Verification items for this drawing (mm, ordinates from the low corner). A direction names the side the tool comes from. Give positions to 0.01 mm unless a question says otherwise; leave off trailing zeros. Order: outer loops, then holes, each group sorted by start corner. A loop starts at its lowest first (then second) coordinate and runs counter-clockwise, first axis right, second up.
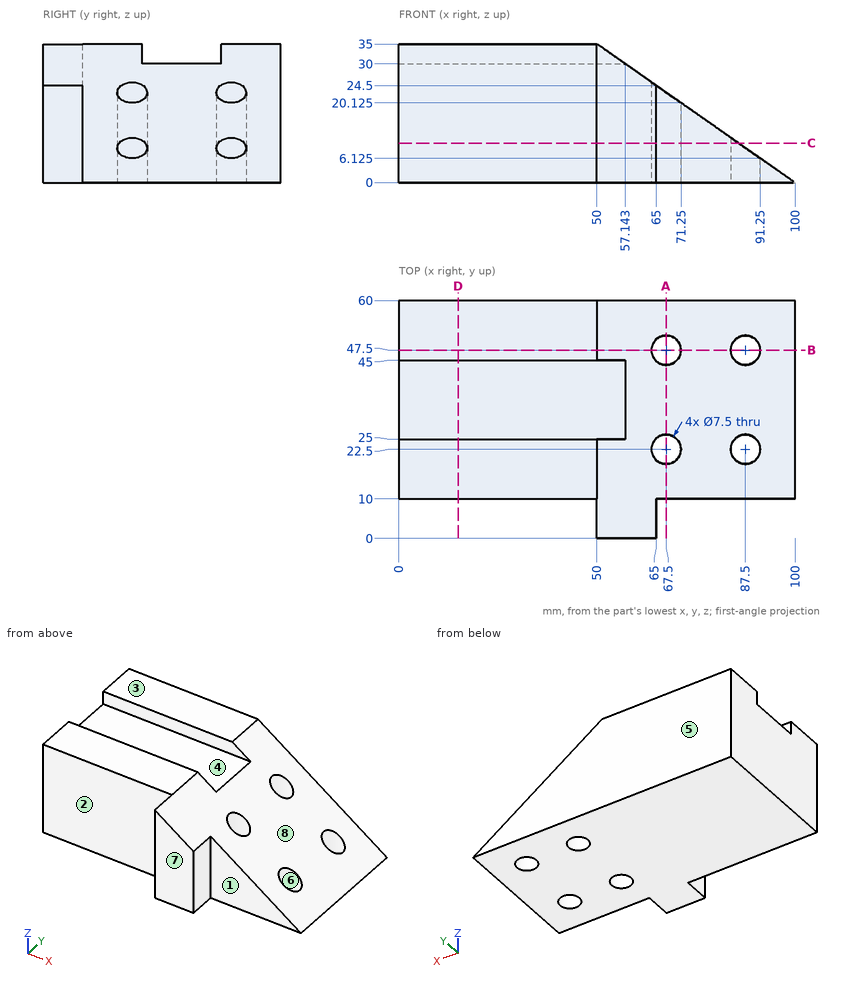
Q1. Cross-section at D-D, the plane x = 15. Record the boundary of the cut face in (y, z), and give its area (3 significant figures).
Q2. Cross-section at B-B, the plane y = 47.5. Record the boundary of the cut face in (x, z) (3 decimals).
Q3. Thickness scan on L1, parallel to Y at x = 67.5, z = 19; L2, parallel to X at y = 22.5, z = 8.25; L3, parallel to Y at x = 44, z = 31. Record the ranges inside material, lowest first.
Q4. Access from +Z, -Z, +X, -X, +Y, -Y to the whole of each face (thin tool, end or side, straight path). Record for the marked faces 1, 2, 3, 4 and 5.
Q5. Release check for a two-part mould opening along X. For the marked faces 6, 7 and 8 record: pulls with the +X half, pulls with the -X half, needs draft (parallel to the pull), parting line crosses it, or undercut.
Q6. Cross-section at A-A, the plane x = 67.5. Record the boundary of the cut face in (y, z).
Q7. Cross-section at C-C, the plane z = 10. Record the boundary of the cut face in (x, y).
Q8. Gauge pin test, flat ends, axial feed: P1, Ø6, axis at x = 28, y = 34, coming from the +Z side; P2, Ø12, axis at x = 67.5, y = 22.5, coming from the +Z side; P3, Ø5, axis at y = 4.5, z = 18.5, coming from the -X side. Record the tip position at first contact, or that the pin passes through.
Answers follow:
1. outline: (10, 0) - (60, 0) - (60, 35) - (45, 35) - (45, 30) - (25, 30) - (25, 35) - (10, 35) - close
1. area: 1,650 mm2
2. outline: (0, 0) - (63.75, 0) - (63.75, 25.375) - (50, 35) - (0, 35) - close; (71.25, 0) - (83.75, 0) - (83.75, 11.375) - (71.25, 20.125) - close; (91.25, 0) - (100, 0) - (91.25, 6.125) - close
3. L1: y = 10 to 18.75, 26.25 to 43.75, 51.25 to 60
3. L2: x = 0 to 63.75, 71.25 to 83.75
3. L3: y = 10 to 25, 45 to 60
4. face 1: +Z, -Z, +X, -Y
4. face 2: +Z, -Z, -X, -Y
4. face 3: +Z, +X, -X, +Y, -Y
4. face 4: +Z, +X, -X
4. face 5: +Z, -Z, +X, -X, +Y
5. face 6: undercut
5. face 7: needs draft
5. face 8: pulls with the +X half
6. outline: (10, 0) - (18.75, 0) - (18.75, 22.75) - (10, 22.75) - close; (26.25, 0) - (43.75, 0) - (43.75, 22.75) - (26.25, 22.75) - close; (51.25, 0) - (60, 0) - (60, 22.75) - (51.25, 22.75) - close
7. outline: (0, 10) - (50, 10) - (50, 0) - (65, 0) - (65, 10) - (85.71, 10) - (85.71, 19.2) arc R3.75 cw to (85.71, 25.8) - (85.71, 44.2) arc R3.75 cw to (85.71, 50.8) - (85.71, 60) - (0, 60) - close; hole circle Ø7.5 at (67.5, 22.5); hole circle Ø7.5 at (67.5, 47.5)
8. P1: stops at z = 30
8. P2: stops at z = 26.95
8. P3: stops at x = 50
